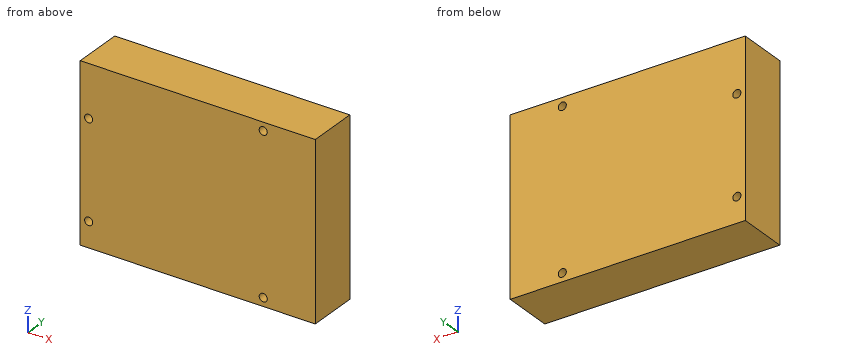
```python
from build123d import *

# Parameters (mm, degrees)
SCHIZZO2_W                   = 70
SCHIZZO2_H                   = 52
ESTRUSIONE_ESTRUSIONE1_DEPTH = 15
FORO_PER_VITE_M2_1_D         = 2.4


with BuildPart() as part:
    # Schizzo2 → Estrusione-Estrusione1 (new body)
    with BuildSketch(Plane(origin=(0, 0, 0), x_dir=(1, 0, 0), z_dir=(0, 1, 0))):
        Rectangle(SCHIZZO2_W, SCHIZZO2_H)
    extrude(amount=ESTRUSIONE_ESTRUSIONE1_DEPTH)

    # Foro per Vite M2-1 (through all)
    with Locations(Plane(origin=(0, 15, 0), x_dir=(1, 0, 0), z_dir=(0, 1, 0))):
        with Locations((19.5, -23.5), (19.5, 23.5), (-32.5, 18.5), (-32.5, -10.5)):
            Hole(FORO_PER_VITE_M2_1_D / 2)


solid = part.part
```
Source: CAD feature listing. Evaluate the final solid. Frame: model axes, mm. Coordinates: 2 decimals unless noted, no trailing zeros. Loops run counter-clockwise (first coordinate to the right, second up) from the corner with the lowest first, then second, coordinate; pieces in that order, holes last. Notation, with made-up numbers: M 16.5,-17 L 24.5,-17 A17 cw 24.5,1 Z; hole C 49.5,-6 d6. An arc over 180 degrees is marked long. Put each result on its own line as item: value. Start each with the question number.
1) Ray query, L1, parallel to Z at x = 19.5, y = 11.25; L2, parallel to Z at x = -32.5, y = 11.5; L3, parallel to X at y = 4.25, z = -23.5. Return the intervals inside material, ascending. Write a range as from..to.
2) Contact query for flat-ended pins moving along their axis: pin 1 Ø4 at (x, z) = (19.5, 23.5) entering from +Y; pin 2 Ø2 at (x, z) = (-32.5, 10.5) entering from +Y. Output: stop coordinate, or through.
3) Cut plane A-A on x = 19.5. Return the cut outline in (y, z).
4) Cut plane B-B on z = -23.5. Return the cut outline in (x, y).
The answers:
1. L1: z = -26..-24.7, -22.3..22.3, 24.7..26
1. L2: z = -26..-19.7, -17.3..9.3, 11.7..26
1. L3: x = -35..18.3, 20.7..35
2. pin 1: stops at y = 15
2. pin 2: passes through
3. outline: M 0,-26 L 15,-26 L 15,-24.7 L 0,-24.7 Z; M 0,-22.3 L 15,-22.3 L 15,22.3 L 0,22.3 Z; M 0,24.7 L 15,24.7 L 15,26 L 0,26 Z
4. outline: M -35,0 L 18.3,0 L 18.3,15 L -35,15 Z; M 20.7,0 L 35,0 L 35,15 L 20.7,15 Z
